The listing builds one solid part. Answer for the finished solid, in the listing's coordinates (mm). A direction names the side the tool comes from. Round coordinates to 2 decimals unless told otherwise and drop trailing zeros. Loops run counter-clockwise (first coordinate to the right, second up) from the corner with the lowest first, then second, coordinate; pieces in that order, holes last. Notation, with made-up numbers: M -16.5,-9 L 27.5,-9 A24 cw 27.5,10 Z; hole C 42.5,66.25 d2. An arc over 180 degrees is marked long. Put each result on its own line as item: value. Start each with the question number.
(1) Section B-B, the plane z = 2.5 is taken. Determine the outline of the cut face in (x, y) (3 decimals), then the cut area to 3 significant figures.
(2) Which of the six approach directions +Z, -Z, +X, -X, +Y, -Y give full straight-line access (tool end or side, diameter ignored) to faces 4 (the face through (22, 29.845, 1)), 5 (the face through (-6, 15, 1.334)), 6 (the face through (19.05, 15, 5)), 7 (the face through (0, 33, 1))?
(3) Flat-ended cylindrical pins translate along their axes: P1, Ø1.9, axis at x = 13, y = 32.5, coming from the +Z side; P2, Ø4, axis at x = 0, z = 4, coming from the -Y side; P3, Ø4, axis at y = 12, z = 7, coming from the -X side; P4, Ø0.7, axis at y = 33, z = 0.5, coming from the +X side. Find the tip coordinate at first contact, or state that the pin passes through.
(4) Section C-C, the plane y = 10 is taken. Count the separate pieces of the cut face and the enclosed holes in it, then the cut area to 3 significant figures.
(5) Section A-A, the plane y = 33.02 is taken. Determine the outline of the cut face in (x, z).
(6) Straight lines are drawn through the part: line 1 (X direction, y = 2, z = 8) (3 decimals); line 2 (X direction, y = 6.5, z = 1.25) (3 decimals); line 3 (Y direction, x = 9.5, z = 5) (3 decimals). For each, find the intervals that lie inside material, in ascending order.
(7) Determine the mould class of faces 1 (the face through (19.05, 33, 1)), 2 (the face through (9, 36.195, 1)), 3 (the face through (9.11, 31.16, 0.28)) for opening direction Y: released by +Y, released by -Y, zero draft, split by the parting line, or undercut.
```python
from build123d import *

# Parameters (mm, degrees)
F1_DEPTH = 8.89
F2_R     = 2.794
F3_DEPTH = 20.32
F0_W     = 6.35
F0_H     = 29.845
F0_R     = 1.905
F0_W_2   = 19.05
F0_H_2   = 6.35
F4_DEPTH = 1.3335
F5_SIZE  = 0.762


with BuildPart() as f1:
    # F0 (on Top) → F1 (new body)
    with BuildSketch(Plane.XY):
        Polygon((0, 29.845), (0, 0), (3.175, 0), (3.175, 26.67), (15.875, 26.67), (15.875, 0), (19.05, 0), (19.05, 29.845), align=None)
    extrude(amount=F1_DEPTH)

    # F2 (on Right) → F3 (cut)
    with BuildSketch(Plane.YZ):
        with Locations((10.795, 4.445)):
            Circle(F2_R)
    extrude(amount=F3_DEPTH, mode=Mode.SUBTRACT)

    # F0 (on Top) → F4 (join)
    with BuildSketch(Plane.XY):
        with Locations((-3.175, 14.9225)):
            Rectangle(F0_W, F0_H)
        with Locations((-3.175, 14.9225)):
            Circle(F0_R, mode=Mode.SUBTRACT)
        with Locations((9.525, 33.02)):
            Rectangle(F0_W_2, F0_H_2)
        with Locations((9.525, 33.02)):
            Circle(F0_R, mode=Mode.SUBTRACT)
        with Locations((22.225, 14.9225)):
            Rectangle(F0_W, F0_H)
        with Locations((22.225, 14.9225)):
            Circle(F0_R, mode=Mode.SUBTRACT)
    extrude(amount=F4_DEPTH)

    # F5
    f5_edges = [f1.edges().sort_by_distance(p)[0] for p in [
        (20.32, 14.9225, 1.3335),
        (-5.08, 14.9225, 1.3335),
        (7.62, 33.02, 1.3335),
    ]]
    chamfer(f5_edges, length=F5_SIZE)


solid = f1.part
```
Recorded:
1. outline: M 0,0 L 3.175,0 L 3.175,8.789 L 0,8.789 Z; M 0,12.801 L 3.175,12.801 L 3.175,26.67 L 15.875,26.67 L 15.875,12.801 L 19.05,12.801 L 19.05,29.845 L 0,29.845 Z; M 15.875,0 L 19.05,0 L 19.05,8.789 L 15.875,8.789 Z
1. area: 204 mm²
2. face 4: +Z, -Z, +X, +Y
2. face 5: +Z, -X, +Y, -Y
2. face 6: +Z, +X, +Y, -Y
2. face 7: +Z, -Z, -X, +Y
3. P1: stops at z = 1.33
3. P2: stops at y = 0
3. P3: stops at x = 0
3. P4: stops at x = 19.05
4. separate pieces: 4
4. enclosed holes: 0
4. area: 39.4 mm²
5. outline: M 0,0 L 7.62,0 L 7.62,0.57 L 6.86,1.33 L 0,1.33 Z; M 11.43,0 L 19.05,0 L 19.05,1.33 L 12.19,1.33 L 11.43,0.57 Z
6. line 1: x = 0 to 3.175, 15.875 to 19.05
6. line 2: x = -6.35 to 3.175, 15.875 to 25.4
6. line 3: y = 26.67 to 29.845
7. face 1: zero draft
7. face 2: released by +Y
7. face 3: undercut
